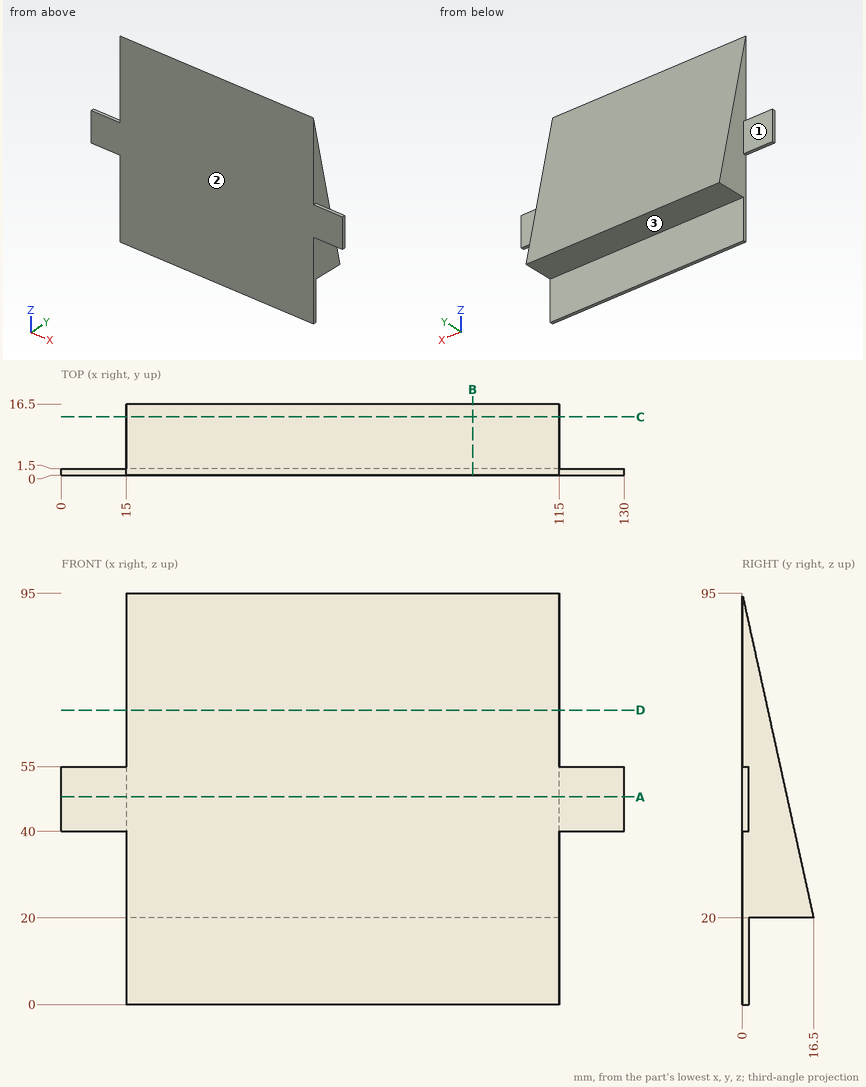
Answer from the drawing. Dimensions are ordinates in mm from the lowest x, y and z of the part. A direction names the side the tool comes from. Give positions to 0.01 mm unless a question says otherwise; leave off trailing zeros. Order: outer loops, then holes, each group sorted by start corner. A loop starts at its lowest first (then second) coordinate and runs counter-clockwise, first axis right, second up. Notation, with made-up numbers: (1, 57.5) -> (15, 57.5) arc R5 ccw to (15, 61.5) -> close; hole circle Ø3 at (63.5, -32). An arc over 180 degrees is marked (long way). Answer as a JSON object with one key per item and string values. Group by question number.
1. Consider line 1 along X through (y, z) = (12.5, 22); line 2 along Y through (x, z) = (100.5, 11); line 3 along Y through (x, z) = (25.5, 45). Determine where each line is inside the solid, lowest interval first. Write a range as [from, to].
2. Section B-B on x = 95 is taken. Determine the outline of the cut face in (y, z), plus the area to 3 significant figures.
3. Section D-D on z = 68 is taken. Determine the outline of the cut face in (x, y).
4. Flat-ended cylindrical pins translate along their axes: pin 1 Ø12 at (x, z) = (98.5, 46.5) entering from +Y; pin 2 Ø1 at (x, y) = (18.5, 7) entering from -Z; pin 3 Ø4.5 at (x, z) = (121, 47) entering from +Y. Find the tip coordinate at first contact, or state that the pin passes through.
5. Section C-C on y = 13.5 is taken. Determine the outline of the cut face in (x, z).
6. Section A-A on z = 48 is taken. Determine the outline of the cut face in (x, y).
7. A tool of negligible diameter and unlimited length cuts with its end or side. For the marked faces 1, 2 and 3, from which of +Z, -Z, +X, -X, +Y, -Y can it reach the whole face along a straight path? Write none if from no direction.
Result sheet:
{
 "1": {"line 1": "x = [15, 115]", "line 2": "y = [0, 1.5]", "line 3": "y = [0, 11]"},
 "2": {"outline": "(0, 0) -> (1.5, 0) -> (1.5, 20) -> (16.5, 20) -> (0, 95) -> close", "area": "649 mm^2"},
 "3": {"outline": "(15, 0) -> (115, 0) -> (115, 5.94) -> (15, 5.94) -> close"},
 "4": {"pin 1": "stops at y = 11.99", "pin 2": "stops at z = 20", "pin 3": "stops at y = 1.5"},
 "5": {"outline": "(15, 20) -> (115, 20) -> (115, 33.64) -> (15, 33.64) -> close"},
 "6": {"outline": "(0, 0) -> (130, 0) -> (130, 1.5) -> (115, 1.5) -> (115, 10.34) -> (15, 10.34) -> (15, 1.5) -> (0, 1.5) -> close"},
 "7": {"face 1": "+Z, -Z, -X, +Y", "face 2": "+Z, -Z, +X, -X, -Y", "face 3": "-Z, +X, -X, +Y"}
}
